CAD build for the part. Positions are in the model's coordinates, mm. Face numbers are marked on the shaded views. A direction names the side the tool comes from. Coordinates: 2 decimals unless noted, no trailing zeros. Order: outer loops, then holes, each group sorted by start corner. A loop starts at its lowest first (then second) coordinate and runs counter-clockwise, first axis right, second up. Notation, with made-up numbers: M 52,54 L 92,54 A14 ccw 92,76 Z; hole C 77.5,44 d8. An arc over 180 degrees is marked long. One line per item, written item: value.
from build123d import *

# Parameters (mm, degrees)
SKETCH1_R           = 110
SKETCH1_R_2         = 100
BOSS_EXTRUDE1_DEPTH = 45
SKETCH2_R           = 110
BOSS_EXTRUDE2_DEPTH = 15
BOSS_EXTRUDE2_TAPER = 60
SKETCH3_R           = 30
BOSS_EXTRUDE3_DEPTH = 100
SKETCH4_R           = 10
SKETCH4_R_2         = 5
CUT_EXTRUDE1_DEPTH  = 100


with BuildPart() as part:
    # Sketch1 → Boss-Extrude1 (new body)
    with BuildSketch(Plane(origin=(0, 0, 0), x_dir=(0, 0, -1), z_dir=(1, 0, 0))):
        with Locations(Location((0, 0, 0), (0, 0, 180))):
            Circle(SKETCH1_R)
        with Locations(Location((0, 0, 0), (0, 0, 180))):
            Circle(SKETCH1_R_2, mode=Mode.SUBTRACT)
    extrude(amount=BOSS_EXTRUDE1_DEPTH)

    # Sketch2 → Boss-Extrude2 (add)
    with BuildSketch(Plane(origin=(45, 0, 0), x_dir=(0, 0, -1), z_dir=(1, 0, 0))):
        with Locations(Location((0, 0, 0), (0, 0, 180))):
            Circle(SKETCH2_R)
    extrude(amount=BOSS_EXTRUDE2_DEPTH, taper=BOSS_EXTRUDE2_TAPER)

    # Sketch3 → Boss-Extrude3 (add)
    with BuildSketch(Plane.ZY.offset(-45)):
        with Locations(Location((0, 0, 0), (0, 0, 180))):
            Circle(SKETCH3_R)
    extrude(amount=BOSS_EXTRUDE3_DEPTH)

    # Sketch4 → Cut-Extrude1 (cut)
    with BuildSketch(Plane(origin=(60, 0, 0), x_dir=(0, 0, -1), z_dir=(1, 0, 0))):
        with Locations((0, 50)):
            Circle(SKETCH4_R)
        with Locations((50, 0)):
            Circle(SKETCH4_R)
        with Locations((0, -50)):
            Circle(SKETCH4_R)
        with Locations((-50, 0)):
            Circle(SKETCH4_R)
        with Locations((35.355339059, 35.355339059)):
            Circle(SKETCH4_R_2)
        with Locations((-35.355339059, -35.355339059)):
            Circle(SKETCH4_R_2)
    extrude(amount=-CUT_EXTRUDE1_DEPTH, mode=Mode.SUBTRACT)


solid = part.part
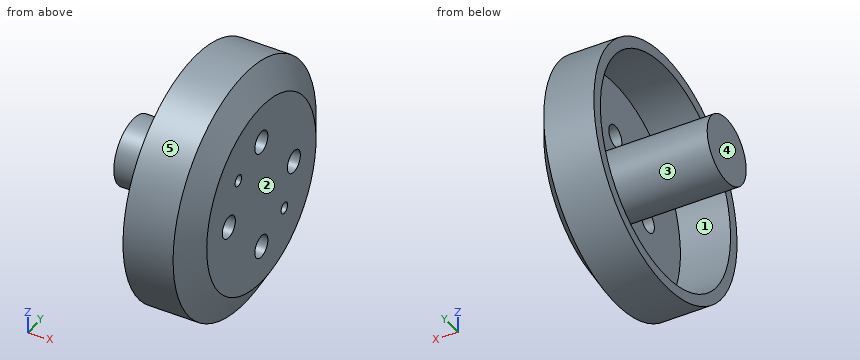
Q1. Mould opens along Z. For the marked faces 3, 4 and 5 say: released by +Z, released by -Z, zero draft, split by the parting line, or undercut.
Recorded:
face 3: undercut
face 4: zero draft
face 5: split by the parting line
Q2. Slice it at A-A (z = 0). List the corners of the cut face in (x, y), plus the area to 3 significant figures.
Recorded:
outline: M -55,-30 L 45,-30 L 45,-40 L 60,-40 L 60,40 L 45,40 L 45,30 L -55,30 Z; M 0,-110 L 45,-110 L 60,-84.02 L 60,-60 L 45,-60 L 45,-100 L 0,-100 Z; M 0,100 L 45,100 L 45,60 L 60,60 L 60,84.02 L 45,110 L 0,110 Z
area: 9,210 mm^2
Q3. Slice it at B-B (x = 52). List the corners of the cut face in (y, z).
Recorded:
outline: C 0,0 d195.75; hole C -50,0 d20; hole C -35.36,35.36 d10; hole C 0,-50 d20; hole C 0,50 d20; hole C 35.36,-35.36 d10; hole C 50,0 d20
Q4. Pin check, flat tips, straight feed: pin 1 Ø2 at (y, z) = (20, 83.5) entering from -X; pin 2 Ø18 at (y, z) = (-50, 0) entering from -X; pin 3 Ø6 at (x, z) = (-25.5, -10.5) entering from +Y; pin 4 Ø1.5 at (y, z) = (-37.5, 81.5) entering from +X. Stop position of each tip, or through.
Recorded:
pin 1: stops at x = 45
pin 2: passes through
pin 3: stops at y = 29.05
pin 4: stops at x = 57.15
Q5. Slice it at C-C (x = 11). List the corners of the cut face in (y, z), plus the area to 3 significant figures.
Recorded:
outline: C 0,0 d220; C 0,0 d60; hole C 0,0 d200
area: 9,420 mm^2
Q6. Which spindle directions (+Z, -Z, +X, -X, +Y, -Y) get a long thin tool onto all of the face, cutting with end or side? Do the marked faces 1 and 2. Say none if no direction does.
Recorded:
face 1: -X
face 2: +Z, -Z, +X, +Y, -Y
Q7. Drill centre lines: line 1 along Y through (x, z) = (17.5, 0); line 2 along Y through (x, z) = (56, 0); line 3 along X through (y, z) = (-18, 41). Where is each one in solid material? Low to high.
Recorded:
line 1: y = -110 to -100, -30 to 30, 100 to 110
line 2: y = -90.95 to -60, -40 to 40, 60 to 90.95
line 3: x = 45 to 60
Q8. Slice it at D-D (y = 0). Give the number of separate pieces and of enclosed holes in the cut face, plus the area to 3 significant figures.
Recorded:
separate pieces: 3
enclosed holes: 0
area: 9,210 mm^2
